Read the model definition and answer for the solid it produces. Units are mm, in the model's axes. A direction names the side the tool comes from. Coordinates: 2 decimals unless noted, no trailing zeros. Loops run counter-clockwise (first coordinate to the right, second up) from the corner with the lowest first, then second, coordinate; pieces in that order, holes last.
from build123d import *
from OCP.BRepFilletAPI import BRepFilletAPI_MakeChamfer

# Parameters (mm, degrees)
SCHIZZO1_R                   = 18.35
ESTRUSIONE_ESTRUSIONE1_DEPTH = 22
SCHIZZO2_R                   = 17.2
ESTRUSIONE_ESTRUSIONE2_DEPTH = 34.6
SCHIZZO3_R                   = 16.55
TAGLIO_ESTRUSIONE1_DEPTH     = 1.5
SCHIZZO4_R                   = 2.75
SCHIZZO4_R_2                 = 3.925
ESTRUSIONE_ESTRUSIONE3_DEPTH = 2
SCHIZZO5_W                   = 0.5
SCHIZZO5_H                   = 2.9
ESTRUSIONE_ESTRUSIONE4_DEPTH = 4.5
SMUSSO1_SIZE                 = 1
SMUSSO1_SIZE2                = 0.577350269
TAGLIO_ESTRUSIONE2_DEPTH     = 71.973886043
SCHIZZO7_R                   = 1.1
TAGLIO_ESTRUSIONE3_DEPTH     = 2
SCHIZZO8_R                   = 1
ESTRUSIONE_ESTRUSIONE5_DEPTH = 4.75
SCHIZZO9_R                   = 1.5
TAGLIO_ESTRUSIONE4_DEPTH     = 5
SCHIZZO10_R                  = 6
ESTRUSIONE_ESTRUSIONE6_DEPTH = 5.85
SCHIZZO11_R                  = 3
ESTRUSIONE_ESTRUSIONE7_DEPTH = 3
ESTRUSIONE_ESTRUSIONE8_DEPTH = 12


with BuildPart() as part:
    # Schizzo1 → Estrusione-Estrusione1 (new body)
    with BuildSketch(Plane(origin=(0, 0, 0), x_dir=(1, 0, 0), z_dir=(0, 1, 0))):
        with Locations(Location((0, 0, 0), (0, 0, 270))):
            Circle(SCHIZZO1_R)
    extrude(amount=ESTRUSIONE_ESTRUSIONE1_DEPTH)

    # Schizzo2 → Estrusione-Estrusione2 (add)
    with BuildSketch(Plane(origin=(0, 22, 0), x_dir=(1, 0, 0), z_dir=(0, 1, 0))):
        with Locations(Location((0, 0, 0), (0, 0, 270))):
            Circle(SCHIZZO2_R)
    extrude(amount=ESTRUSIONE_ESTRUSIONE2_DEPTH)

    # Schizzo3 → Taglio-Estrusione1 (cut)
    with BuildSketch(Plane(origin=(0, 56.6, 0), x_dir=(1, 0, 0), z_dir=(0, 1, 0))):
        with Locations(Location((0, 0, 0), (0, 0, 270))):
            Circle(SCHIZZO3_R)
    extrude(amount=-TAGLIO_ESTRUSIONE1_DEPTH, mode=Mode.SUBTRACT)

    # Schizzo4 → Estrusione-Estrusione3 (add)
    with BuildSketch(Plane(origin=(0, 55.1, 0), x_dir=(1, 0, 0), z_dir=(0, 1, 0))):
        with Locations(Location((11.5, 0, 0), (0, 0, 270))):
            Circle(SCHIZZO4_R)
        with Locations(Location((-11.5, 0, 0), (0, 0, 270))):
            Circle(SCHIZZO4_R)
        with Locations(Location((0, 0, 0), (0, 0, 270))):
            Circle(SCHIZZO4_R_2)
    extrude(amount=ESTRUSIONE_ESTRUSIONE3_DEPTH)

    # Schizzo5 → Estrusione-Estrusione4 (add)
    with BuildSketch(Plane(origin=(0, 57.1, 0), x_dir=(1, 0, 0), z_dir=(0, 1, 0))):
        with Locations((-11.5, 0)):
            Rectangle(SCHIZZO5_W, SCHIZZO5_H)
        with Locations((11.5, 0)):
            Rectangle(SCHIZZO5_W, SCHIZZO5_H)
    extrude(amount=ESTRUSIONE_ESTRUSIONE4_DEPTH)

    # Smusso1: one chamfer whose edges measure the first distance from different faces: ONE call of the kernel's chamfer builder (chamfer() names one face for all edges)
    smusso1_edges_1 = [part.edges().sort_by_distance(p)[0] for p in [
        (-11.5, 61.6, -1.45),
    ]]
    smusso1_side_1 = [part.faces().sort_by_distance(p)[0] for p in [
        (-11.5, 59.35, -1.45),
    ]]
    smusso1_edges_2 = [part.edges().sort_by_distance(p)[0] for p in [
        (-11.5, 61.6, 1.45),
    ]]
    smusso1_side_2 = [part.faces().sort_by_distance(p)[0] for p in [
        (-11.5, 59.35, 1.45),
    ]]
    smusso1_edges_3 = [part.edges().sort_by_distance(p)[0] for p in [
        (11.5, 61.6, -1.45),
    ]]
    smusso1_side_3 = [part.faces().sort_by_distance(p)[0] for p in [
        (11.5, 59.35, -1.45),
    ]]
    smusso1_edges_4 = [part.edges().sort_by_distance(p)[0] for p in [
        (11.5, 61.6, 1.45),
    ]]
    smusso1_side_4 = [part.faces().sort_by_distance(p)[0] for p in [
        (11.5, 59.35, 1.45),
    ]]
    smusso1 = BRepFilletAPI_MakeChamfer(part.part.solid().wrapped)
    for e in smusso1_edges_1:
        smusso1.Add(SMUSSO1_SIZE, SMUSSO1_SIZE2, e.wrapped, smusso1_side_1[0].wrapped)  # the first distance lies on this face
    for e in smusso1_edges_2:
        smusso1.Add(SMUSSO1_SIZE, SMUSSO1_SIZE2, e.wrapped, smusso1_side_2[0].wrapped)  # the first distance lies on this face
    for e in smusso1_edges_3:
        smusso1.Add(SMUSSO1_SIZE, SMUSSO1_SIZE2, e.wrapped, smusso1_side_3[0].wrapped)  # the first distance lies on this face
    for e in smusso1_edges_4:
        smusso1.Add(SMUSSO1_SIZE, SMUSSO1_SIZE2, e.wrapped, smusso1_side_4[0].wrapped)  # the first distance lies on this face
    add(Compound.cast(smusso1.Shape()), mode=Mode.REPLACE)

    # Schizzo6 → Taglio-Estrusione2 (cut, through all)
    with BuildSketch(Plane.ZY.offset(11.75)):
        with BuildLine():
            Line((0.675, 59.95), (0.675, 57.95))
            ThreePointArc((0.675, 57.95), (0, 57.275), (-0.675, 57.95))
            Line((-0.675, 57.95), (-0.675, 59.95))
            ThreePointArc((-0.675, 59.95), (0, 60.625), (0.675, 59.95))
        make_face()
    extrude(amount=-TAGLIO_ESTRUSIONE2_DEPTH, mode=Mode.SUBTRACT)

    # Schizzo7 → Taglio-Estrusione3 (cut)
    with BuildSketch(Plane(origin=(0, 57.1, 0), x_dir=(1, 0, 0), z_dir=(0, 1, 0))):
        with Locations(Location((0, 0, 0), (0, 0, 270))):
            Circle(SCHIZZO7_R)
    extrude(amount=-TAGLIO_ESTRUSIONE3_DEPTH, mode=Mode.SUBTRACT)

    # Schizzo8 → Estrusione-Estrusione5 (add)
    with BuildSketch(Plane(origin=(0, 55.1, 0), x_dir=(1, 0, 0), z_dir=(0, 1, 0))):
        with Locations(Location((0, 0, 0), (0, 0, 270))):
            Circle(SCHIZZO8_R)
    extrude(amount=ESTRUSIONE_ESTRUSIONE5_DEPTH)

    # Schizzo9 → Taglio-Estrusione4 (cut)
    with BuildSketch(Plane.XZ):
        with Locations(Location((0, -15.5, 0), (0, 0, 270))):
            Circle(SCHIZZO9_R)
        with Locations(Location((-13.423393759, -7.75, 0), (0, 0, 270))):
            Circle(SCHIZZO9_R)
        with Locations(Location((-13.423393759, 7.75, 0), (0, 0, 270))):
            Circle(SCHIZZO9_R)
        with Locations(Location((0, 15.5, 0), (0, 0, 270))):
            Circle(SCHIZZO9_R)
        with Locations(Location((13.423393759, 7.75, 0), (0, 0, 270))):
            Circle(SCHIZZO9_R)
        with Locations(Location((13.423393759, -7.75, 0), (0, 0, 270))):
            Circle(SCHIZZO9_R)
    extrude(amount=-TAGLIO_ESTRUSIONE4_DEPTH, mode=Mode.SUBTRACT)

    # Schizzo10 → Estrusione-Estrusione6 (add)
    with BuildSketch(Plane.XZ):
        with Locations(Location((-6.65, 0, 0), (0, 0, 270))):
            Circle(SCHIZZO10_R)
    extrude(amount=ESTRUSIONE_ESTRUSIONE6_DEPTH)

    # Schizzo11 → Estrusione-Estrusione7 (add)
    with BuildSketch(Plane.XZ.offset(5.85)):
        with Locations(Location((-6.65, 0, 0), (0, 0, 270))):
            Circle(SCHIZZO11_R)
    extrude(amount=ESTRUSIONE_ESTRUSIONE7_DEPTH)

    # Schizzo12 → Estrusione-Estrusione8 (add)
    with BuildSketch(Plane.XZ.offset(8.85)):
        with BuildLine():
            ThreePointArc((-9.65, 0), (-7.598683298, -2.846049894), (-4.25, -1.8))
            Line((-4.25, -1.8), (-4.25, 0))
            Line((-4.25, 0), (-9.65, 0))
        make_face()
        with BuildLine():
            Line((-9.65, 0), (-4.25, 0))
            Line((-4.25, 0), (-4.25, 1.8))
            ThreePointArc((-4.25, 1.8), (-7.598683298, 2.846049894), (-9.65, 0))
        make_face()
    extrude(amount=ESTRUSIONE_ESTRUSIONE8_DEPTH)


solid = part.part
Q1. A cutting plane is placed at B-B (x = -6.65). Give the vertices of the cut face in (y, z), then the cut area to 3 significant figures.
Findings below:
outline: (-20.85, -3) - (-5.85, -3) - (-5.85, -6) - (0, -6) - (0, -17.1) - (22, -17.1) - (22, -15.86) - (56.6, -15.86) - (56.6, -15.16) - (55.1, -15.16) - (55.1, 15.16) - (56.6, 15.16) - (56.6, 15.86) - (22, 15.86) - (22, 17.1) - (0, 17.1) - (0, 6) - (-5.85, 6) - (-5.85, 3) - (-20.85, 3) - close
area: 1,960 mm2
Q2. Straight lines are drawn through the part: probe 1 along Y at (x, z) = (-6, -15.5); probe 2 along Y at (x, z) = (14, 6); probe 3 along X at (y, z) = (1, 7). For each, find the intervals that lie inside material, in ascending order.
Findings below:
probe 1: y = 0 to 56.6
probe 2: y = 0 to 55.1
probe 3: x = -16.96 to -14.72, -12.12 to 12.12, 14.72 to 16.96
Q3. A cutting plane is placed at C-C (y = 19). Give the vertices of the cut face in (x, z).
Findings below:
outline: circle Ø36.7 at (0, 0)
Q4. A cutting plane is placed at D-D (y = 40). Give the vertices of the cut face in (x, z).
Findings below:
outline: circle Ø34.4 at (0, 0)
Q5. A cutting plane is placed at A-A (z = 15.5). Give the vertices of the cut face in (x, y), then the cut area to 3 significant figures.
Findings below:
outline: (-9.82, 0) - (-1.5, 0) - (-1.5, 5) - (1.5, 5) - (1.5, 0) - (9.82, 0) - (9.82, 22) - (7.46, 22) - (7.46, 56.6) - (5.8, 56.6) - (5.8, 55.1) - (-5.8, 55.1) - (-5.8, 56.6) - (-7.46, 56.6) - (-7.46, 22) - (-9.82, 22) - close
area: 916 mm2
Q6. Determine the mould class of faces 1 (the face through (14.1, 56.6, -9)), 2 (the face through (-3, 55.1, 3)), 3 (the face through (-10.466, 39.058, -13.649)) for opening direction X: +X half, -X half, draft (parallel to the pull), parting line (faces both ways), or undercut.
Findings below:
face 1: draft
face 2: undercut
face 3: parting line
Q7. Which of the six approach directions +Z, -Z, +X, -X, +Y, -Y give full straight-line access (tool end or side, diameter ignored) to faces 4 (the face through (11.25, 59, 1)), 5 (the face through (-12.41, 2.465, 8.856)), 6 (the face through (14.227, 56.086, -0.358))?
Findings below:
face 4: +Z, -Z, +Y
face 5: -Y
face 6: +Y
Q8. Flat-ended cylindrical pins translate along their axes: pin 1 Ø0.9 at (x, z) = (13.5, -7.5) entering from -Y; pin 2 Ø6 at (x, y) = (-9.5, -5.5) entering from -Z; pin 3 Ø5 at (x, z) = (0, -15.5) entering from -Y. Find the tip coordinate at first contact, or state that the pin passes through.
Findings below:
pin 1: stops at y = 5
pin 2: stops at z = -6
pin 3: stops at y = 0
